from build123d import *

# Parameters (mm, degrees)
F0_W      = 96
F0_H      = 78
F1_DEPTH  = 18
F2_W      = 72
F2_H      = 38
F4_DEPTH  = 58
F6_DEPTH  = 38
F7_W      = 8
F7_H      = 12
F8_DEPTH  = 60.001
F10_DEPTH = 72.001
F11_W     = 20
F11_H     = 5
F12_DEPTH = 96.001
F13_W     = 46
F13_H     = 26
F14_DEPTH = 5
F17_DEPTH = 23.001
F18_W     = 3
F18_H     = 14
F19_DEPTH = 72
F20_R     = 2.99999


# Not quite as in the source:
# - a fillet or chamfer is up to 0.001 mm smaller than in the source, because OpenCascade refuses the exact size


with BuildPart() as f1:
    # F0 (on Top) → F1 (new body)
    with BuildSketch(Plane.XY):
        with Locations((48, 39)):
            Rectangle(F0_W, F0_H)
    extrude(amount=F1_DEPTH)

    # F2 (on face) → F4 (join, through all)
    with BuildSketch(Plane.XY.offset(18)):
        with Locations((48, 59)):
            Rectangle(F2_W, F2_H)
    extrude(amount=F4_DEPTH)

    # F5 (on face) → F6 (cut, through all)
    with BuildSketch(Plane(origin=(0, 78, 0), x_dir=(-1, 0, 0), z_dir=(0, 1, 0))):
        Polygon((-60, 76), (-84, 76), (-84, 52), align=None)
    extrude(amount=-F6_DEPTH, mode=Mode.SUBTRACT)

    # F7 (on face) → F8 (cut, through all)
    with BuildSketch(Plane(origin=(12, 0, 0), x_dir=(0, -1, 0), z_dir=(-1, 0, 0))):
        with Locations((-52, 70)):
            Rectangle(F7_W, F7_H)
    extrude(amount=-F8_DEPTH, mode=Mode.SUBTRACT)

    # F9 (on face) → F10 (cut, through all)
    with BuildSketch(Plane(origin=(12, 0, 0), x_dir=(0, -1, 0), z_dir=(-1, 0, 0))):
        Polygon((-78, 40), (-64, 76), (-78, 76), align=None)
    extrude(amount=-F10_DEPTH, mode=Mode.SUBTRACT)

    # F11 (on face) → F12 (cut, through all)
    with BuildSketch(Plane.YZ.offset(96)):
        with Locations((20, 2.5)):
            Rectangle(F11_W, F11_H)
    extrude(amount=-F12_DEPTH, mode=Mode.SUBTRACT)

    # F13 (on face) → F14 (join)
    with BuildSketch(Plane.XY.offset(18)):
        with BuildLine():
            Line((25, 7), (25, 33))
            ThreePointArc((25, 33), (12, 20), (25, 7))
        make_face()
        with BuildLine():
            ThreePointArc((71, 7), (84, 20), (71, 33))
            Line((71, 33), (71, 7))
        make_face()
        with Locations((48, 20)):
            Rectangle(F13_W, F13_H)
    extrude(amount=F14_DEPTH)

    # F15 (on face) → F17 (cut, through all)
    with BuildSketch(Plane.XY.offset(23)):
        with BuildLine():
            ThreePointArc((25, 26), (19, 20), (25, 14))
            Line((25, 14), (71, 14))
            ThreePointArc((71, 14), (77, 20), (71, 26))
            Line((71, 26), (25, 26))
        make_face()
    extrude(amount=-F17_DEPTH, mode=Mode.SUBTRACT)

    # F18 (on face) → F19 (cut, through all)
    with BuildSketch(Plane.YZ.offset(84)):
        with Locations((41.5, 25)):
            Rectangle(F18_W, F18_H)
    extrude(amount=-F19_DEPTH, mode=Mode.SUBTRACT)

    # F20 (radius 3 in the source; OpenCascade refuses exactly that, so slightly less here)
    f20_edges = [f1.edges().sort_by_distance(p)[0] for p in [
        (48, 7, 18),
        (48, 43, 18),
        (48, 43, 32),
        (48, 0, 18),
        (0, 39, 18),
        (84, 60.5, 18),
        (12, 60.5, 18),
        (96, 39, 18),
        (96, 0, 9),
        (0, 0, 9),
        (96, 78, 9),
        (0, 78, 9),
    ]]
    fillet(f20_edges, radius=F20_R)


solid = f1.part
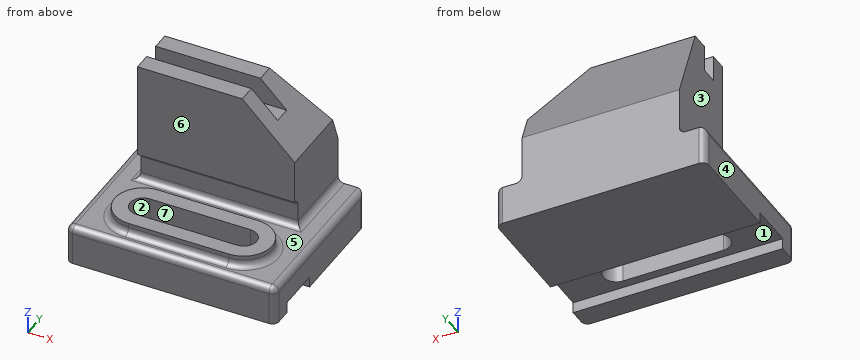
Build history of the part. All positions in model axes, mm. Face numbers are marked on the shaded views. A direction names the side the tool comes from. Coordinates: 2 decimals unless noted, no trailing zeros. Write each loop counter-clockwise with the first axis right and the second up, starting at its lowest first coordinate (ties: lowest second). Pieces come first, ordered by that corner, then holes.
(1) Cut at C-C on y = 60. List the corners of the cut face in (x, z), and give its area (3 significant figures).
(2) 3-axis set-ups, long thin cutter, end or side, ignore diameter. For the marked faces 1, 2 and 3: which of +Z, -Z, +X, -X, +Y, -Y reach the whole face in a straight line?
(3) Cut at A-A on y = 20. List the corners of the cut face in (x, z), and give its area (3 significant figures).
(4) Mould opens along Y. For the marked faces 4, 5, 6 and 7 say: pulls with the +Y half, pulls with the -Y half, needs draft (parallel to the pull), parting line crosses it, or undercut.
(5) Pin check, flat tips, straight feed: pin 1 Ø1 at (x, z) = (39.5, 22.5) entering from -Y; pin 2 Ø3 at (y, z) = (57.5, 28) entering from -X; pin 3 Ø4 at (y, z) = (40, 45) entering from +X; pin 4 Ø9 at (x, z) = (38, 18) entering from -Y. Stop position of each tip, or through.
(6) Drill centre lines: line 1 (Y direction, x = 58.5, z = 19.5); line 2 (Y direction, x = 43, z = 11.5); line 3 (Z direction, x = 14, y = 18). Where is each one in solid material? Low to high.
Working result:
1. outline: (0, 0) - (96, 0) - (96, 15) arc R3 ccw to (93, 18) - (87, 18) arc R3 cw to (84, 21) - (84, 52) - (60, 76) - (12, 76) - (12, 21) arc R3 cw to (9, 18) - (3, 18) arc R3 ccw to (0, 15) - close
1. area: 5,620 mm2
2. face 1: -Z, +X, -X
2. face 2: +Z, -Z
2. face 3: +Z, -X, +Y, -Y
3. outline: (0, 5) - (19, 5) - (19, 23) - (12, 23) - (12, 21) arc R3 cw to (9, 18) - (3, 18) arc R3 ccw to (0, 15) - close; (77, 5) - (96, 5) - (96, 15) arc R3 ccw to (93, 18) - (87, 18) arc R3 cw to (84, 21) - (84, 23) - (77, 23) - close
3. area: 564 mm2
4. face 4: needs draft
4. face 5: undercut
4. face 6: pulls with the -Y half
4. face 7: undercut
5. pin 1: stops at y = 7
5. pin 2: stops at x = 12
5. pin 3: stops at x = 84
5. pin 4: stops at y = 0
6. line 1: y = 6.6 to 14, 26 to 33.4, 42.6 to 78
6. line 2: y = 0 to 14, 26 to 78
6. line 3: z = 5 to 23
